from build123d import *

# Parameters (mm, degrees)
SKETCH1_R           = 18.5
BOSS_EXTRUDE1_DEPTH = 59.8
SKETCH2_R           = 6
SKETCH2_R_2         = 3
BOSS_EXTRUDE2_DEPTH = 5
BOSS_EXTRUDE3_DEPTH = 14
SKETCH2_5_R         = 1.5
CUT_EXTRUDE1_DEPTH  = 5


with BuildPart() as part:
    # Sketch1 → Boss-Extrude1 (new body)
    with BuildSketch(Plane(origin=(0, 0, 0), x_dir=(1, 0, 0), z_dir=(0, 1, 0))):
        Circle(SKETCH1_R)
    extrude(amount=BOSS_EXTRUDE1_DEPTH)

    # Sketch2 → Boss-Extrude2 (add)
    with BuildSketch(Plane(origin=(0, 59.8, 0), x_dir=(1, 0, 0), z_dir=(0, 1, 0))):
        Circle(SKETCH2_R)
        Circle(SKETCH2_R_2, mode=Mode.SUBTRACT)
        with BuildLine():
            ThreePointArc((1.658312395, 2.5), (0, 3), (-1.658312395, 2.5))
            Line((-1.658312395, 2.5), (1.658312395, 2.5))
        make_face()
        with BuildLine():
            Line((1.658312395, 2.5), (-1.658312395, 2.5))
            ThreePointArc((-1.658312395, 2.5), (-1.418637165, -2.643382037), (3, 0))
            ThreePointArc((3, 0), (2.643382037, 1.418637165), (1.658312395, 2.5))
        make_face()
    extrude(amount=BOSS_EXTRUDE2_DEPTH)

    # Sketch2_3 → Boss-Extrude3 (add)
    with BuildSketch(Plane(origin=(0, 59.8, 0), x_dir=(1, 0, 0), z_dir=(0, 1, 0))):
        with BuildLine():
            Line((1.658312395, 2.5), (-1.658312395, 2.5))
            ThreePointArc((-1.658312395, 2.5), (-1.418637165, -2.643382037), (3, 0))
            ThreePointArc((3, 0), (2.643382037, 1.418637165), (1.658312395, 2.5))
        make_face()
    extrude(amount=BOSS_EXTRUDE3_DEPTH)

    # Sketch2_5 → Cut-Extrude1 (cut)
    with BuildSketch(Plane(origin=(0, 59.8, 0), x_dir=(1, 0, 0), z_dir=(0, 1, 0))):
        with Locations((-13.423393759, 7.75)):
            Circle(SKETCH2_5_R)
        with Locations((0, 15.5)):
            Circle(SKETCH2_5_R)
        with Locations((13.423393759, 7.75)):
            Circle(SKETCH2_5_R)
        with Locations((13.423393759, -7.75)):
            Circle(SKETCH2_5_R)
        with Locations((0, -15.5)):
            Circle(SKETCH2_5_R)
        with Locations((-13.423393759, -7.75)):
            Circle(SKETCH2_5_R)
    extrude(amount=-CUT_EXTRUDE1_DEPTH, mode=Mode.SUBTRACT)


solid = part.part
Geometry check sheet. Reference: the model listing, model coordinates, mm. A direction names the side the tool comes from. Coordinates: 2 decimals unless noted, no trailing zeros. Order: outer loops, then holes, each group sorted by start corner. A loop starts at its lowest first (then second) coordinate and runs counter-clockwise, first axis right, second up. Notation, with made-up numbers: (74, 59.5) - (90, 59.5) arc R20 ccw to (90, 63.5) - close; hole circle Ø11 at (-23, -29). An arc over 180 degrees is marked (long way). Answer in a Markdown table with one row per item. Add a question column.
1) Cross-section at D-D, the plane y = 68.5. Record the cut outline in (x, z), then the cut area to 3 significant figures.
2) Gauge pin test, flat ends, axial feed: P1, Ø3, axis at x = 0, y = 55, coming from the +Z side; P2, Ø2.5, axis at x = 0, z = -15.5, coming from the +Y side; P3, Ø8, axis at x = 5.5, y = 49.5, coming from the -Z side. Record the tip position at first contact, or that the pin passes through.
3) Cross-section at B-B, the plane x = 0. Record the cut outline in (y, z), then the cut area to 3 significant figures.
4) Release check for a two-part mould opening along X. For faces 1 (the cylindrical face through (-6, 62, 0)), 2 (the cylindrical face through (12.23, 57.33, 8.66)), 3 (the flat face through (-4.4, 59.8, -4.4)), 4 (the cylindrical face through (-1.11, 57.33, -16.51)) record: +X half, -X half, draft (parallel to the pull), parting line (faces both ways), or undercut.
5) Cross-section at A-A, the plane y = 56.5. Record the cut outline in (x, z).
6) Set-up check for faces 5 (the flat face through (0, 69, -2.5)), 6 (the flat face through (0, 73.8, 0)), 7 (the flat face through (0, 54.8, 15)): record each of +Z, -Z, +X, -X, +Y, -Y from which the full face is reachable in a straight line by a thin tool's end or side.
7) Cross-section at C-C, the plane z = -15.5. Record the cut outline in (x, y), then the cut area to 3 significant figures.
8) Material ranges on line 1 along Z through (x, y) = (0, 58.15); line 2 along X through (y, z) = (57, 7); line 3 along Y through (x, z) = (-11.5, 0.5), recorded low to high. Write a range as [from, to].
Check result:
| question | item | result |
|---|---|---|
| 1 | outline | (-1.66, -2.5) - (1.66, -2.5) arc R3 ccw (long way) to start |
| 1 | area | 27.1 mm² |
| 2 | P1 | stops at z = 18.5 |
| 2 | P2 | stops at y = 54.8 |
| 2 | P3 | stops at z = -18.44 |
| 3 | outline | (0, -18.5) - (59.8, -18.5) - (59.8, -17) - (54.8, -17) - (54.8, -14) - (59.8, -14) - (59.8, -6) - (64.8, -6) - (64.8, -2.5) - (73.8, -2.5) - (73.8, 3) - (64.8, 3) - (64.8, 6) - (59.8, 6) - (59.8, 14) - (54.8, 14) - (54.8, 17) - (59.8, 17) - (59.8, 18.5) - (0, 18.5) - close |
| 3 | area | 2,290 mm² |
| 4 | face 1 | parting line |
| 4 | face 2 | undercut |
| 4 | face 3 | draft |
| 4 | face 4 | undercut |
| 5 | outline | circle Ø37 at (0, 0); hole circle Ø3 at (-13.42, -7.75); hole circle Ø3 at (-13.42, 7.75); hole circle Ø3 at (0, -15.5); hole circle Ø3 at (0, 15.5); hole circle Ø3 at (13.42, -7.75); hole circle Ø3 at (13.42, 7.75) |
| 6 | face 5 | -Z, +X, -X, +Y |
| 6 | face 6 | +Z, -Z, +X, -X, +Y |
| 6 | face 7 | +Y |
| 7 | outline | (-10.1, 0) - (10.1, 0) - (10.1, 59.8) - (1.5, 59.8) - (1.5, 54.8) - (-1.5, 54.8) - (-1.5, 59.8) - (-10.1, 59.8) - close |
| 7 | area | 1,190 mm² |
| 8 | line 1 | z = [-18.5, -17], [-14, 14], [17, 18.5] |
| 8 | line 2 | x = [-17.12, -14.72], [-12.12, 12.12], [14.72, 17.12] |
| 8 | line 3 | y = [0, 59.8] |
